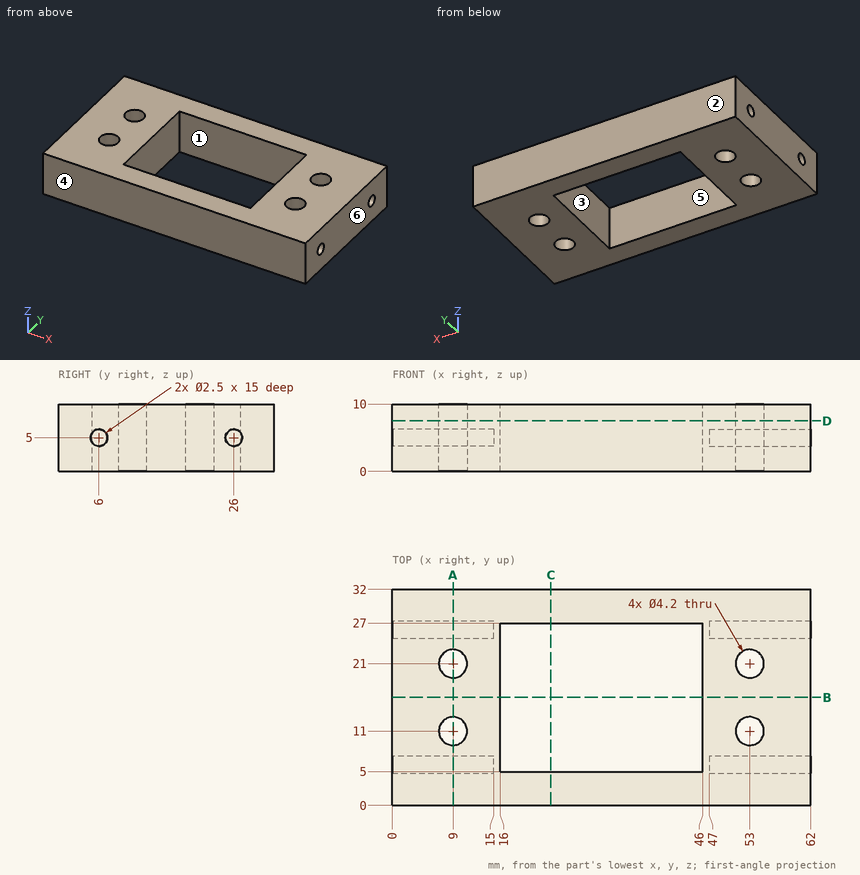
Check sheet for the drawn part. Datum: minimum x, y, z corner. Units: mm. A direction names the side the tool comes from. Coordinates: 2 decimals unless noted, no trailing zeros. Order: outer loops, then holes, each group sorted by start corner. A loop starts at its lowest first (then second) coordinate and runs counter-clockwise, first axis right, second up. Notation, with made-up numbers: (54.5, 86) -> (112.5, 86) arc R21 ccw to (112.5, 112) -> close; hole circle Ø1 at (-38, -37.5). An arc over 180 degrees is marked (long way). Write each question's results on one line, items separated by ' | '. Start each with the question number.
1) Depth check by flat-ended pin: pin 1 (2.5 mm diameter, centred on x = 53, y = 11, fed in from +Z); pin 2 (2 mm diameter, centred on y = 6, z = 5, fed in from +X). Enter the tip coordinate at first touch or a pass-through.
2) Section check A-A (x = 9). Enter the section's corners in (y, z).
3) Section check C-C (x = 23.5). Enter the section's corners in (y, z).
4) Section check D-D (z = 7.5). Enter the section's corners in (x, y).
5) Draft check along Y on the marked faces 1, 2, 3 and 4. Enter one of: pulls with the +Y half, pulls with the -Y half, needs draft (parallel to the pull), parting line crosses it, or undercut.
6) Set-up check for the marked faces 5 and 6: record each of +Z, -Z, +X, -X, +Y, -Y from which the full face is reachable in a straight line by a thin tool's end or side.
7) Material ranges on line 1 along Y through (x, z) = (9, 7.75); line 2 along X through (y, z) = (6, 2.75); line 3 along Z through (x, y) = (50.75, 26), recorded low to high.
8) Section check B-B (y = 16). Enter the section's corners in (x, z), and give its area (3 significant figures).
Checked values:
1) pin 1: through | pin 2: x = 47
2) outline: (0, 0) -> (8.9, 0) -> (8.9, 10) -> (0, 10) -> close; (13.1, 0) -> (18.9, 0) -> (18.9, 10) -> (13.1, 10) -> close; (23.1, 0) -> (32, 0) -> (32, 10) -> (23.1, 10) -> close; hole circle Ø2.5 at (6, 5); hole circle Ø2.5 at (26, 5)
3) outline: (0, 0) -> (5, 0) -> (5, 10) -> (0, 10) -> close; (27, 0) -> (32, 0) -> (32, 10) -> (27, 10) -> close
4) outline: (0, 0) -> (62, 0) -> (62, 32) -> (0, 32) -> close; hole circle Ø4.2 at (9, 11); hole circle Ø4.2 at (9, 21); hole (16, 5) -> (46, 5) -> (46, 27) -> (16, 27) -> close; hole circle Ø4.2 at (53, 11); hole circle Ø4.2 at (53, 21)
5) face 1: undercut | face 2: pulls with the +Y half | face 3: undercut | face 4: pulls with the -Y half
6) face 5: +Z, -Z | face 6: +Z, -Z, +X, +Y, -Y
7) line 1: 0 to 8.9, 13.1 to 18.9, 23.1 to 32 | line 2: 0 to 16, 46 to 62 | line 3: 0 to 3.75, 6.25 to 10
8) outline: (0, 0) -> (16, 0) -> (16, 10) -> (0, 10) -> close; (46, 0) -> (62, 0) -> (62, 10) -> (46, 10) -> close | area: 320 mm²
